Can you work these out from the model? Positions are in its coordinate system, mm. Face numbers are marked on the shaded views. A direction names the side the tool comes from. Coordinates: 2 decimals unless noted, no trailing zeros. Order: outer loops, then holes, each group sorted by start corner. A loop starts at its lowest first (then second) coordinate and runs counter-clockwise, first axis right, second up. Notation, with made-up numbers: (0, 64) -> (39, 64) arc R12 ccw to (39, 70) -> close; hole circle Ø6 at (28, -34.75). An arc over 180 degrees is marked (long way). Use a Markdown table: item, result. Add a question column.
1. We'd pull the mould along X, two halves only. Please class the marked faces 5, 6 and 7: pulls with the +X half, pulls with the -X half, needs draft (parallel to the pull), parting line crosses it, or undercut.
2. Suppose I cut it at C-C, the plane y = -50.38. List the corners of the cut face in (x, z) for me.
3. For pin 1 Ø16 at (y, z) = (-18.5, 26.5) entering from +X; pin 2 Ø5.5 at (y, z) = (-30, 22) entering from -X; pin 3 Ø8.5 at (x, y) = (-20, -50.38) entering from -Z; pin 4 Ø9 at (x, y) = (20.5, -12.5) entering from +Z, each with a flat end and sliding along its axis, tell me the tip position at first contact or that it passes through.
4. Suppose I cut it at D-D, the plane x = 0. List the corners of the cut face in (y, z) for me, then the cut area to 3 significant figures.
5. For the marked faces 1, 2, 3 and 4, which set-ups out of +Z, -Z, +X, -X, +Y, -Y let a thin tool reach every point of the face, with its end or its side?
6. If I drill on line 1 along Y through (x, z) = (3.25, 22); line 2 along Y through (x, z) = (15, 7); line 3 along X through (y, z) = (-13.5, 21.5), over which ranges is the centre line in solid material (lowest first)? Write a range as from..to.
7. Suppose I cut it at B-B, the plane z = 22. List the corners of the cut face in (x, y) for me.
8. Suppose I cut it at A-A, the plane x = -30. List the corners of the cut face in (y, z) for me, then the cut area to 3 significant figures.
Autodesk Inventor part; units mm, degrees
ref_plane "YZ Plane" through (0, 0, 0) normal (1, 0, 0) x (0, 1, 0)
ref_plane "XZ Plane" through (0, 0, 0) normal (0, 1, 0) x (-1, 0, 0)
ref_plane "XY Plane" through (0, 0, 0) normal (0, 0, 1) x (1, 0, 0)
sketch "Sketch1" plane through (0, 0, 0) normal (0, 0, 1) x (1, 0, 0)
  circle A0 centre (0, 0) radius 37.5
  line L0 (0, 0) -> (0, -25)
  circle A1 centre (0, -25) radius 3
  dimension "d0" = 75
  dimension "d1" = 25
  dimension "d2" = 6
extrude "Extrusion1" add sketch "Sketch1" along normal blind 8 contours A0 | A1
sketch "Sketch2" plane through (0, 0, 8) normal (0, 0, 1) x (1, 0, 0)
  line L0 (0, 0) -> (17.6777, 17.6777)
  line L1 (0, 0) -> (25, 0) construction
  circle A0 centre (17.6777, 17.6777) radius 3.15
  circle A1 centre (-17.6777, 17.6777) radius 3.15
  circle A2 centre (-17.6777, -17.6777) radius 3.15
  circle A3 centre (17.6777, -17.6777) radius 3.15
  dimension "d5" = 25
  dimension "d6" = 45
  dimension "d7" = 6.3
  dimension "d10" = 360
extrude "Extrusion2" cut sketch "Sketch2" against normal blind 10
sketch "Sketch3" plane through (0, 0, 8) normal (0, 0, 1) x (1, 0, 0)
  arc A0 (-21.9203, 13.435) -> (-13.435, 21.9203) centre (-17.6777, 17.6777) ccw
  line L0 (-17.6777, 17.6777) -> (-11.6777, 17.6777) construction
  line L1 (-13.435, 21.9203) -> (-19.9189, 28.4042)
  line L2 (-21.9203, 13.435) -> (-28.4042, 19.9189)
  line L3 (-28.4042, 19.9189) -> (-19.9189, 28.4042)
  arc A1 (-13.435, -21.9203) -> (-21.9203, -13.435) centre (-17.6777, -17.6777) ccw
  line L4 (-17.6777, -17.6777) -> (-17.6777, -11.6777) construction
  line L5 (-21.9203, -13.435) -> (-28.4042, -19.9189)
  line L6 (-13.435, -21.9203) -> (-19.9189, -28.4042)
  line L7 (-19.9189, -28.4042) -> (-28.4042, -19.9189)
  arc A2 (21.9203, -13.435) -> (13.435, -21.9203) centre (17.6777, -17.6777) ccw
  line L8 (17.6777, -17.6777) -> (11.6777, -17.6777) construction
  line L9 (13.435, -21.9203) -> (19.9189, -28.4042)
  line L10 (21.9203, -13.435) -> (28.4042, -19.9189)
  line L11 (28.4042, -19.9189) -> (19.9189, -28.4042)
  arc A3 (13.435, 21.9203) -> (21.9203, 13.435) centre (17.6777, 17.6777) ccw
  line L12 (17.6777, 17.6777) -> (17.6777, 11.6777) construction
  line L13 (21.9203, 13.435) -> (28.4042, 19.9189)
  line L14 (13.435, 21.9203) -> (19.9189, 28.4042)
  line L15 (19.9189, 28.4042) -> (28.4042, 19.9189)
  circle A4 centre (0, 0) radius 31.5
  point P0 (-26.1087, 17.6234)
  point P1 (-26.1087, -17.6234)
  point P2 (-17.6234, -26.1087)
  point P3 (17.6234, -26.1087)
  point P4 (26.1087, -17.6234)
  point P5 (26.1087, 17.6234)
  point P6 (17.6234, 26.1087)
  point P7 (-17.6234, 26.1087)
  dimension "d14" = 12
  dimension "d18" = 360
sketch "Sketch4" plane through (0, 0, 0) normal (0, 0, -1) x (-1, 0, 0)
  circle A0 centre (0, 0) radius 42.8826
extrude "Extrusion4" cut sketch "Sketch4" against normal blind 2
sketch "Sketch5" plane through (0, 0, 8) normal (0, 0, 1) x (1, 0, 0)
  line L0 (0, 0) -> (8, 0)
  line L1 (8, 0) -> (8, -40)
  line L2 (8, -40) -> (-8, -40)
  line L3 (-8, -40) -> (-8, 40)
  line L4 (-8, 40) -> (8, 40)
  line L5 (8, 40) -> (8, -40)
  line L6 (0, 0) -> (0, 8)
  line L7 (0, 8) -> (40, 8)
  line L8 (40, 8) -> (40, -8)
  line L9 (40, -8) -> (-40, -8)
  line L10 (-40, -8) -> (-40, 8)
  line L11 (-40, 8) -> (40, 8)
  line L12 (0, 0) -> (0, 40)
  line L13 (0, 40) -> (-5, 40)
  line L14 (-5, 40) -> (5, 40)
  line L15 (5, 40) -> (5, -40)
  line L16 (5, -40) -> (-5, -40)
  line L17 (-5, -40) -> (-5, 40)
  point P0 (8, -8)
  point P1 (8, 8)
  point P2 (-8, 8)
  point P3 (-8, -8)
  dimension "d24" = 8
  dimension "d25" = 40
  dimension "d26" = 16
  dimension "d27" = 80
  dimension "d30" = 90
  dimension "d34" = 5
  dimension "d35" = 10
sketch "Sketch6" plane through (0, 0, 8) normal (0, 0, 1) x (1, 0, 0)
  line L0 (0, 0) -> (0, 40)
  line L1 (0, 40) -> (-5, 40)
  line L2 (-5, 40) -> (5, 40)
  line L3 (5, 40) -> (5, -40)
  line L4 (5, -40) -> (-5, -40)
  line L5 (-5, -40) -> (-5, 40)
  line L6 (0, 0) -> (-40, 0)
  line L7 (-40, 0) -> (-40, -5)
  line L8 (-40, -5) -> (-40, 5)
  line L9 (-40, 5) -> (40, 5)
  line L10 (40, 5) -> (40, -5)
  line L11 (40, -5) -> (-40, -5)
  circle A0 centre (0, 0) radius 37.5
  point P0 (5, -5)
  point P1 (5, 5)
  point P2 (-5, 5)
  point P3 (-5, -5)
  point P4 (37.1652, 5)
  point P5 (5, 37.1652)
  point P6 (-5, 37.1652)
  point P7 (-37.1652, 5)
  point P8 (-37.1652, -5)
  point P9 (-5, -37.1652)
  point P10 (5, -37.1652)
  point P11 (37.1652, -5)
  dimension "d36" = 40
  dimension "d37" = 5
  dimension "d38" = 10
  dimension "d39" = 80
  dimension "d42" = 90
  dimension "d46" = 75
extrude "Extrusion7" add sketch "Sketch6" along normal blind 30 contours L6 L5 L9 L0 | L0 L9 L3 L11 L5 L6 | L9 L5 A0 L0 | L0 A0 L3 L9 | L6 A0 L9 L5 | L5 L11 A0 L6 | L9 A0 L11 L3 | L11 L3 A0 L5
sketch "Sketch7" plane through (5, 5, 8) normal (0, 1, 0) x (1, 0, 0)
  line L0 (0, 0) -> (0, -30)
  line L1 (0, 0) -> (-5, 0)
  line L2 (-5, 0) -> (25, 0)
  line L3 (0, 0) -> (32.1652, 0)
  line L4 (25, 0) -> (25, -14)
  circle A0 centre (25, -14) radius 1.65
  point P0 (-5, 8)
  dimension "d49" = 5
  dimension "d50" = 30
  dimension "d51" = 14
  dimension "d52" = 3.3
extrude "Extrusion8" cut sketch "Sketch7" against normal blind 20
ref_plane "Work Plane1" through (5, 0, 8) normal (0, 1, 0) x (1, 0, 0)
ref_plane "Work Plane2" through (0, 5, 8) normal (1, 0, 0) x (0, 0, -1)
pattern_circular "Circular Pattern2" count 2 over 90 about axis through (0, 0, 8) along (0, 0, 1) of "Extrusion8"
sketch "Sketch8" plane through (-37.1652, 5, 8) normal (0, 1, 0) x (1, 0, 0)
  line L0 (32.1652, 0) -> (32.1652, -30)
  line L1 (32.1652, 0) -> (37.1652, 0)
  line L2 (37.1652, 0) -> (5.9902, 0)
  line L3 (22.6375, 0) -> (16.3375, 0)
  line L4 (5.9902, 0) -> (5.9902, -14)
  circle A0 centre (5.9902, -14) radius 2.15
  point P0 (37.1652, 8)
  dimension "d61" = 31.175
  dimension "d62" = 14
  dimension "d63" = 4.3
extrude "Extrusion9" [suppressed]
pattern_circular "Circular Pattern3" count 2 over 360 about axis through (0, 0, 8) along (0, 0, -1) of "Extrusion8"
sketch "Sketch10" plane through (5, 5, 8) normal (1, 0, 0) x (0, 0, -1)
  line L0 (0, 0) -> (-30, 0)
  line L1 (0, 0) -> (-30, 0)
  line L2 (-30, 0) -> (-30, 35.3175)
  line L3 (-30, 35.3175) -> (0, 35.3175)
  line L4 (0, 35.3175) -> (0, 0)
  line L5 (0, -10) -> (-30, -10)
  line L6 (0, -10) -> (-32.3439, -10)
  line L7 (-32.3439, -10) -> (-32.3439, -45.8466)
  line L8 (-32.3439, -45.8466) -> (0, -45.8466)
  line L9 (0, -45.8466) -> (0, -10)
  point P0 (8, -5)
extrude "Extrusion11" cut sketch "Sketch10" against normal blind 0.12
mirror "Mirror2" about plane through (0, 5, 8) normal (1, 0, 0) of "Extrusion11"
sketch "Sketch11" plane through (37.1652, 5, 38) normal (0, 1, 0) x (1, 0, 0)
  line L0 (-32.2852, 30) -> (-32.2852, 0)
  line L1 (-32.2852, 30) -> (5.1404, 30)
  line L2 (5.1404, 30) -> (5.1404, -1.2125)
  line L3 (5.1404, -1.2125) -> (-32.2852, -1.2125)
  line L4 (-32.2852, -1.2125) -> (-32.2852, 30)
  line L5 (-74.3303, 30) -> (-42.0452, 30)
  line L6 (-42.0452, 30) -> (-76.613, 30)
  line L7 (-76.613, 30) -> (-76.613, -1.2125)
  line L8 (-76.613, -1.2125) -> (-42.0452, -1.2125)
  line L9 (-42.0452, -1.2125) -> (-42.0452, 30)
  point P0 (-37.1652, 38)
extrude "Extrusion12" cut sketch "Sketch11" against normal blind 0.12
mirror "Mirror3" about plane through (5, 0, 8) normal (0, 1, 0) of "Extrusion12"
mirror "Mirror4" about plane through (5, 0, 8) normal (0, 1, 0) of "Extrusion8", "Circular Pattern2"
chamfer "Chamfer4" distance 3 angle 45 8 edges at (21.0306, 4.88, 38) (-21.0306, 4.88, 38) (4.88, -21.0306, 38) (4.88, 21.0306, 38) (-4.88, -21.0306, 38) (-4.88, 21.0306, 38) (21.0306, -4.88, 38) (-21.0306, -4.88, 38)
sketch "Sketch13" plane through (0, 0, 8) normal (0, 0, 1) x (1, 0, 0)
  arc A0 (37.1811, 4.88) -> (4.88, 37.1811) centre (0, 0) ccw
  circle A1 centre (0, 0) radius 37.5
  line L0 (37.1811, 4.88) -> (4.88, 4.88)
  line L1 (4.88, 4.88) -> (4.88, 37.1811)
  line L2 (37.1811, 4.88) -> (4.88, 4.88)
  line L3 (4.88, 4.88) -> (4.88, 37.1811)
  line L4 (4.88, 37.1811) -> (37.1811, 37.1811)
  line L5 (37.1811, 37.1811) -> (37.1811, 4.88)
  circle A2 centre (17.6777, 17.6777) radius 3.15
  circle A3 centre (17.6777, 17.6777) radius 6
  line L6 (0, 0) -> (0, 7.2893)
  line L7 (0, 0) -> (7.7636, 0)
  arc A4 (-4.88, 37.1811) -> (-37.1811, 4.88) centre (0, 0) ccw
  circle A5 centre (0, 0) radius 37.5
  line L8 (-37.1811, 4.88) -> (-4.88, 4.88)
  line L9 (-4.88, 4.88) -> (-4.88, 37.1811)
  line L10 (-37.1811, 4.88) -> (-4.88, 4.88)
  line L11 (-4.88, 4.88) -> (-4.88, 37.1811)
  line L12 (-4.88, 37.1811) -> (-37.1811, 37.1811)
  line L13 (-37.1811, 37.1811) -> (-37.1811, 4.88)
  circle A6 centre (-17.6777, 17.6777) radius 3.15
  circle A7 centre (-17.6777, 17.6777) radius 6
  arc A8 (4.88, -37.1811) -> (37.1811, -4.88) centre (0, 0) ccw
  circle A9 centre (0, 0) radius 37.5
  line L14 (37.1811, -4.88) -> (4.88, -4.88)
  line L15 (4.88, -4.88) -> (4.88, -37.1811)
  line L16 (37.1811, -4.88) -> (4.88, -4.88)
  line L17 (4.88, -4.88) -> (4.88, -37.1811)
  line L18 (4.88, -37.1811) -> (37.1811, -37.1811)
  line L19 (37.1811, -37.1811) -> (37.1811, -4.88)
  circle A10 centre (17.6777, -17.6777) radius 3.15
  circle A11 centre (17.6777, -17.6777) radius 6
  line L20 (0, 0) -> (0, -7.2893)
  arc A12 (-37.1811, -4.88) -> (-4.88, -37.1811) centre (0, 0) ccw
  circle A13 centre (0, 0) radius 37.5
  line L21 (-37.1811, -4.88) -> (-4.88, -4.88)
  line L22 (-4.88, -4.88) -> (-4.88, -37.1811)
  line L23 (-37.1811, -4.88) -> (-4.88, -4.88)
  line L24 (-4.88, -4.88) -> (-4.88, -37.1811)
  line L25 (-4.88, -37.1811) -> (-37.1811, -37.1811)
  line L26 (-37.1811, -37.1811) -> (-37.1811, -4.88)
  circle A14 centre (-17.6777, -17.6777) radius 3.15
  circle A15 centre (-17.6777, -17.6777) radius 6
  arc A16 (1.88, 37.4528) -> (-1.88, 37.4528) centre (0, 0) ccw
  line L27 (1.88, 37.4528) -> (-1.88, 37.4528)
  line L28 (4.88, 37.1811) -> (17.88, 37.1811)
  line L29 (4.88, 37.1811) -> (4.88, 24.0161)
  point P0 (-37.1811, -4.88)
  dimension "d96" = 12
  dimension "d97" = 13
  dimension "d98" = 13.165
extrude "Extrusion14" add sketch "Sketch13" along normal blind 7 contours L0 L1 A0 | A1 L15 L14 | L9 L8 A1 | A1 L21 L22
sketch "Sketch19" plane through (0, 0, 2) normal (0, 0, -1) x (-1, 0, 0)
  circle A0 centre (-17.6777, 17.6777) radius 3.15
  circle A1 centre (-17.6777, 17.6777) radius 9.67
  circle A2 centre (17.6777, 17.6777) radius 3.15
  circle A3 centre (17.6777, 17.6777) radius 9.0628
  circle A4 centre (17.6777, -17.6777) radius 3.15
  circle A5 centre (17.6777, -17.6777) radius 10.6824
  circle A6 centre (-17.6777, -17.6777) radius 3.15
  circle A7 centre (-17.6777, -17.6777) radius 10.6824
  point P0 (0, 0)
extrude "Extrusion19" add sketch "Sketch19" against normal blind 13 contours A0 | A1 | A2 | A3 | A4 | A5 | A6 | A7
sketch "Sketch21" plane through (0, 0, 2) normal (0, 0, -1) x (-1, 0, 0)
  circle A0 centre (0, 0) radius 37.5
  line L0 (-37.5, 0) -> (37.5, 0)
  line L1 (37.5, 0) -> (37.5, -60)
  line L2 (37.5, -60) -> (-37.5, -60)
  line L3 (-37.5, -60) -> (-37.5, 0)
  dimension "d145" = 75
  dimension "d146" = 60
extrude "Extrusion22" add sketch "Sketch21" against normal blind 13 contours L1 L2 L3 A0
sketch "Sketch22" plane through (0, 0, 15) normal (0, 0, 1) x (1, 0, 0)
  line L0 (0, 0) -> (20, 0)
  line L1 (20, 0) -> (20, -4.88)
  line L2 (4.88, -4.88) -> (37.1811, -4.88)
  line L3 (20, -4.88) -> (20, -10.38)
  line L4 (0, 0) -> (-20, 0)
  line L5 (-20, 0) -> (-20, -4.88)
  line L6 (-37.1811, -4.88) -> (-4.88, -4.88)
  line L7 (-20, -4.88) -> (-20, -10.38)
  line L8 (-20, -10.38) -> (20, -10.38)
  line L9 (20, -10.38) -> (20, -50.38)
  line L10 (20, -50.38) -> (-20, -50.38)
  line L11 (-20, -50.38) -> (-20, -10.38)
  circle A0 centre (-20, -50.38) radius 2.65
  circle A1 centre (-20, -10.38) radius 2.65
  circle A2 centre (20, -10.38) radius 2.65
  circle A3 centre (20, -50.38) radius 2.65
  dimension "d149" = 20
  dimension "d150" = 5.5
  dimension "d151" = 20
  dimension "d152" = 5.5
  dimension "d153" = 40
  dimension "d154" = 40
  dimension "d155" = 5.3
  dimension "d156" = 5.3
  dimension "d157" = 5.3
  dimension "d158" = 5.3
extrude "Extrusion23" cut sketch "Sketch22" against normal blind 13 contours A2 L9 L3 | L3 L8 A2 | A1 L8 L7 | L7 L11 A1 | L9 A2 L8 | L8 A1 L11 | A0 L10 L11 | L11 L10 A0 | A3 L10 L9 | L9 L10 A3
sketch "Sketch23" plane through (0, 0, 15) normal (0, 0, 1) x (1, 0, 0)
  circle A0 centre (-20, -10.38) radius 2.65
  circle A1 centre (-20, -10.38) radius 5.5
  line L0 (-37.1811, -4.88) -> (-4.88, -4.88)
  circle A2 centre (20, -10.38) radius 2.65
  circle A3 centre (20, -10.38) radius 5.5
  circle A4 centre (20, -50.38) radius 2.65
  circle A5 centre (20, -50.38) radius 5.5
  circle A6 centre (-20, -50.38) radius 2.65
  circle A7 centre (-20, -50.38) radius 5.5
  point P0 (0, 0)
  dimension "d161" = 11
  dimension "d162" = 11
extrude "Extrusion24" cut sketch "Sketch23" against normal blind 9 contours A0 | A1 | A3 | A4 | A5 | A6 | A7
properties part number "Test_Stand_Mounting_Plate"
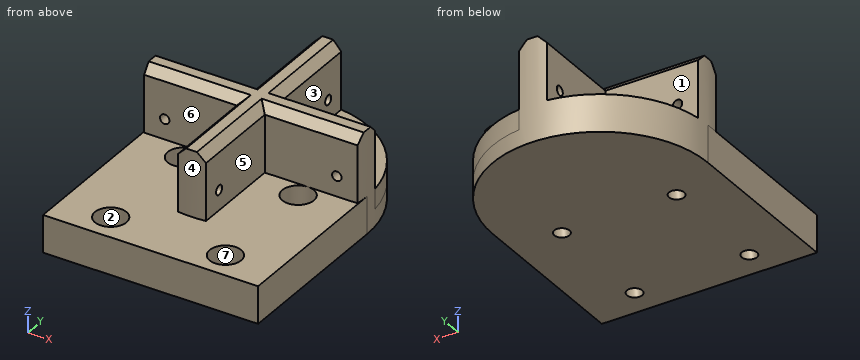
Worked out:
| question | item | result |
|---|---|---|
| 1 | face 5 | pulls with the +X half |
| 1 | face 6 | needs draft |
| 1 | face 7 | undercut |
| 2 | outline | (-37.5, 2) -> (-22.65, 2) -> (-22.65, 6) -> (-25.5, 6) -> (-25.5, 15) -> (-37.5, 15) -> close; (-17.35, 2) -> (17.35, 2) -> (17.35, 6) -> (14.5, 6) -> (14.5, 15) -> (-14.5, 15) -> (-14.5, 6) -> (-17.35, 6) -> close; (22.65, 2) -> (37.5, 2) -> (37.5, 15) -> (25.5, 15) -> (25.5, 6) -> (22.65, 6) -> close |
| 3 | pin 1 | stops at x = 4.88 |
| 3 | pin 2 | stops at x = -4.88 |
| 3 | pin 3 | stops at z = 2 |
| 3 | pin 4 | stops at z = 15 |
| 4 | outline | (-60, 2) -> (37.5, 2) -> (37.5, 38) -> (-37.5, 38) -> (-37.5, 15) -> (-60, 15) -> close; hole circle Ø3.3 at (-30, 22); hole circle Ø3.3 at (30, 22) |
| 4 | area | 2,980 mm² |
| 5 | face 1 | +Z, -X, +Y |
| 5 | face 2 | +Z |
| 5 | face 3 | +Z, +X, +Y |
| 5 | face 4 | +Z, -Y |
| 6 | line 1 | y = -37.36..-31.65, -28.35..28.35, 31.65..37.36 |
| 6 | line 2 | y = -60..-52.67, -48.09..-12.67, -8.09..34.37 |
| 6 | line 3 | x = -4.88..4.88 |
| 7 | outline | (-37.18, -4.88) -> (-31.65, -4.88) -> (-31.65, 4.88) -> (-37.18, 4.88) arc R37.5 ccw to start; (-28.35, -4.88) -> (-4.88, -4.88) -> (-4.88, -28.35) -> (4.88, -28.35) -> (4.88, -4.88) -> (28.35, -4.88) -> (28.35, 4.88) -> (4.88, 4.88) -> (4.88, 28.35) -> (-4.88, 28.35) -> (-4.88, 4.88) -> (-28.35, 4.88) -> close; (-4.88, -37.18) arc R37.5 ccw to (4.88, -37.18) -> (4.88, -31.65) -> (-4.88, -31.65) -> close; (-4.88, 31.65) -> (4.88, 31.65) -> (4.88, 37.18) arc R37.5 ccw to (-4.88, 37.18) -> close; (31.65, -4.88) -> (37.18, -4.88) arc R37.5 ccw to (37.18, 4.88) -> (31.65, 4.88) -> close |
| 8 | outline | (-60, 2) -> (22.5, 2) -> (22.5, 15) -> (4.88, 15) -> (4.88, 20.35) -> (-4.88, 20.35) -> (-4.88, 15) -> (-60, 15) -> close; (-4.88, 23.65) -> (4.88, 23.65) -> (4.88, 35) -> (1.88, 38) -> (-1.88, 38) -> (-4.88, 35) -> close |
| 8 | area | 1,260 mm² |
